Check sheet for the modelled part. Datum: model origin and axes. Units: mm. Face numbers are marked on the shaded views. Give positions to 0.01 mm unless a question says otherwise; leave off trailing zeros. Loops run counter-clockwise (first coordinate to the right, second up) from the corner with the lowest first, then second, coordinate; pieces in that order, holes last. Notation, with made-up numbers: M 42.5,4 L 87.5,4 A22 cw 87.5,40 Z; hole C 85,47 d8. An arc over 180 degrees is marked long. Use one line per item in the form item = value.
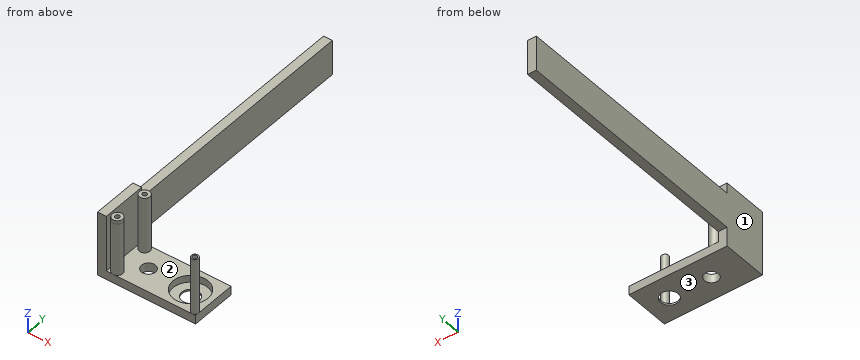
Autodesk Inventor part; units mm, degrees
ref_plane "YZ Plane" through (0, 0, 0) normal (1, 0, 0) x (0, 1, 0)
ref_plane "XZ Plane" through (0, 0, 0) normal (0, 1, 0) x (-1, 0, 0)
ref_plane "XY Plane" through (0, 0, 0) normal (0, 0, 1) x (1, 0, 0)
sketch "Sketch1" plane through (0, 0, 0) normal (0, 0, 1) x (1, 0, 0)
  line L0 (0, 0) -> (50.8, 0)
  line L1 (50.8, 0) -> (50.8, -33.02)
  line L2 (50.8, -33.02) -> (0, -33.02)
  line L3 (0, -33.02) -> (0, 0)
  dimension "d0" = 50.8
  dimension "d1" = 33.02
extrude "Extrusion1" add sketch "Sketch1" along normal blind 6.35
sketch "Sketch2" plane through (0, 0, 6.35) normal (0, 0, 1) x (1, 0, 0)
  line L0 (50.8, 0) -> (0, 0)
  line L1 (0, 0) -> (0, -33.02)
  circle A0 centre (34.29, -16.51) radius 12.7
  point P0 (7.62, -16.51)
  dimension "d4" = 16.51
  dimension "d5" = 16.51
  dimension "d6" = 26.67
  dimension "d7" = 7.62
  dimension "d8" = 25.4
extrude "Extrusion2" cut sketch "Sketch2" against normal blind 5.08
sketch "Sketch3" plane through (34.29, -16.51, 1.27) normal (0, 0, 1) x (1, 0, 0)
  circle A0 centre (0, 0) radius 6.35
  point P0 (-34.29, 16.51)
  dimension "d11" = 12.7
extrude "Extrusion3" cut sketch "Sketch3" against normal blind 5.08
sketch "Sketch14" plane through (0, -33.02, 0) normal (-1, 0, 0) x (0, 0, 1)
  line L0 (0, 33.02) -> (6.35, 33.02)
  line L1 (6.35, 33.02) -> (6.35, 0)
  line L2 (6.35, 0) -> (0, 0)
  line L3 (0, 0) -> (0, 33.02)
extrude "Extrusion14" add sketch "Sketch14" along normal blind 12.7
sketch "Sketch15" plane through (0, 0, 6.35) normal (0, 0, 1) x (1, 0, 0)
  line L0 (-12.7, -33.02) -> (-12.7, 0)
  line L1 (50.8, -33.02) -> (-12.7, -33.02)
  line L2 (50.8, 0) -> (-12.7, 0)
  circle A0 centre (-8.89, -3.81) radius 3.81
  circle A1 centre (-8.89, -29.21) radius 3.81
  circle A2 centre (-8.89, -29.21) radius 1.651
  circle A3 centre (-8.89, -3.81) radius 1.651
  point P0 (0, 0)
  dimension "d58" = 3.81
  dimension "d59" = 3.81
  dimension "d60" = 3.81
  dimension "d61" = 3.81
  dimension "d62" = 7.62
  dimension "d63" = 7.62
  dimension "d64" = 3.302
  dimension "d65" = 3.302
extrude "Extrusion15" add sketch "Sketch15" along normal blind 38.1 contours A1 | A0
sketch "Sketch16" plane through (0, 0, 6.35) normal (0, 0, 1) x (1, 0, 0)
  circle A0 centre (48.26, -30.48) radius 2.54
  line L0 (50.8, -33.02) -> (-8.89, -33.02)
  line L1 (50.8, -33.02) -> (50.8, 0)
  circle A1 centre (48.26, -30.48) radius 1.651
  point P0 (0, 0)
  dimension "d68" = 5.08
  dimension "d69" = 2.54
  dimension "d70" = 2.54
  dimension "d71" = 3.302
extrude "Extrusion16" add sketch "Sketch16" along normal blind 38.1 contours A0
sketch "Sketch17" plane through (-8.89, -3.81, 44.45) normal (0, 0, 1) x (1, 0, 0)
  circle A0 centre (0, 0) radius 1.651
  circle A1 centre (0, 0) radius 1.651
  circle A2 centre (0, 0) radius 3.81
  circle A3 centre (0, -25.396) radius 1.651
  circle A4 centre (0, -25.396) radius 3.81
  circle A5 centre (57.15, -26.67) radius 1.651
  circle A6 centre (57.15, -26.67) radius 1.651
  circle A7 centre (57.15, -26.67) radius 2.54
  point P0 (8.89, 3.81)
  dimension "d74" = 3.302
  dimension "d75" = 7.62
  dimension "d76" = 3.302
  dimension "d77" = 7.62
  dimension "d78" = 5.08
extrude "Extrusion17" add sketch "Sketch17" along normal blind 2.54
sketch "Sketch18" plane through (-12.7, -33.02, 0) normal (-1, 0, 0) x (0, 0, 1)
  line L0 (6.35, 3.81) -> (6.35, 0)
  line L1 (0, 33.02) -> (6.35, 33.02)
  line L2 (6.35, 33.02) -> (6.35, 0)
  line L3 (6.35, 0) -> (0, 0)
  line L4 (0, 0) -> (0, 33.02)
extrude "Extrusion18" add sketch "Sketch18" along normal blind 12.7
sketch "Sketch20" plane through (-25.4, -33.02, 0) normal (-1, 0, 0) x (0, 0, 1)
  line L0 (0, 33.02) -> (0, 0)
  line L1 (0, 0) -> (6.35, 0)
  line L2 (0, 33.02) -> (6.35, 33.02)
  line L3 (6.35, 33.02) -> (6.35, 0)
  line L4 (6.35, 0) -> (0, 0)
  line L5 (0, 0) -> (0, 33.02)
extrude "Extrusion20" cut sketch "Sketch20" against normal blind 5.08
sketch "Sketch21" plane through (0, 0, 6.35) normal (0, 0, 1) x (1, 0, 0)
  line L0 (-20.32, 0) -> (50.8, 0)
  line L1 (-20.32, 0) -> (-13.97, 0)
  line L2 (-13.97, 0) -> (-13.97, -33.02)
  line L3 (-13.97, -33.02) -> (-20.32, -33.02)
  line L4 (-20.32, -33.02) -> (-20.32, 0)
  point P0 (0, 0)
  dimension "d88" = 6.35
  dimension "d89" = 33.02
extrude "Extrusion21" add sketch "Sketch21" along normal blind 40.64
sketch "Sketch23" plane through (50.8, 0, 6.35) normal (0, 1, 0) x (1, 0, 0)
  line L0 (-64.77, 0) -> (-64.77, -40.64)
  line L1 (-64.77, -7.62) -> (-71.12, -7.62)
  line L2 (-71.12, -7.62) -> (-71.12, -33.02)
  line L3 (-71.12, -33.02) -> (-64.77, -33.02)
  line L4 (-64.77, -33.02) -> (-64.77, -7.62)
  line L5 (-64.77, -40.64) -> (-71.12, -40.64)
  point P0 (-50.8, 6.35)
  dimension "d94" = 25.4
  dimension "d95" = 6.35
  dimension "d96" = 7.62
extrude "Extrusion23" add sketch "Sketch23" along normal blind 177.8
sketch "Sketch24" plane through (0, 0, 6.35) normal (0, 0, 1) x (1, 0, 0)
  circle A0 centre (3.81, -16.51) radius 5.08
  circle A1 centre (34.29, -16.51) radius 6.35
  line L0 (48.26, -33.02) -> (-8.89, -33.02)
  point P0 (0, 0)
  dimension "d99" = 10.16
  dimension "d100" = 30.48
  dimension "d101" = 16.51
extrude "Extrusion24" cut sketch "Sketch24" against normal blind 25.4 contours A0
properties part number "servo attachment claw"
1) Section check A-A (x = 3.81). Record the cut outline in (y, z), then the cut area to 3 significant figures.
Evaluation:
outline = M -33.02,0 L -21.59,0 L -21.59,6.35 L -33.02,6.35 Z; M -11.43,0 L 0,0 L 0,6.35 L -11.43,6.35 Z
area = 145 mm^2
2) Scan lines: line 1 (X direction, y = -16, z = 3); line 2 (Y direction, x = 48.26, z = 16); line 3 (Y direction, x = -8, z = 45). Record each from-to range of solid material in increasing order.
Evaluation:
line_1 = -20.32 to -1.24, 8.86 to 21.6, 46.98 to 50.8
line_2 = -33.02 to -32.13, -28.83 to -27.94
line_3 = -32.91 to -30.6, -27.82 to -25.5, -7.51 to -5.2, -2.42 to -0.11
3) Section check B-B (z = 20.5). Record the cut outline in (x, y).
Evaluation:
outline = M -20.32,-33.02 L -13.97,-33.02 L -13.97,177.8 L -20.32,177.8 Z; C -8.89,-29.21 d7.62; C -8.89,-3.81 d7.62; C 48.26,-30.48 d5.08; hole C -8.89,-29.21 d3.3; hole C -8.89,-3.81 d3.3; hole C 48.26,-30.48 d3.3
4) Depth check by flat-ended pin: pin 1 Ø1 at (x, y) = (-9, -28.5) entering from +Z; pin 2 Ø8 at (x, y) = (3.81, -16.51) entering from +Z; pin 3 Ø5 at (x, y) = (-15.5, 63.5) entering from +Z; pin 4 Ø7 at (x, z) = (1, 9) entering from +Y. Enter the tip coordinate at first touch or a pass-through.
Evaluation:
pin_1 = 6.35
pin_2 = through
pin_3 = 39.37
pin_4 = 0
5) Release check for a two-part mould opening along X. For the marked faces 1, 2 and 3 record: pulls with the +X half, pulls with the -X half, needs draft (parallel to the pull), parting line crosses it, or undercut.
Evaluation:
face_1 = pulls with the -X half
face_2 = undercut
face_3 = needs draft
6) Section check C-C (y = -16.51). Record the cut outline in (x, z), then the cut area to 3 significant figures.
Evaluation:
outline = M -20.32,0 L -1.27,0 L -1.27,6.35 L -13.97,6.35 L -13.97,46.99 L -20.32,46.99 Z; M 8.89,0 L 27.94,0 L 27.94,1.27 L 21.59,1.27 L 21.59,6.35 L 8.89,6.35 Z; M 40.64,0 L 50.8,0 L 50.8,6.35 L 46.99,6.35 L 46.99,1.27 L 40.64,1.27 Z
area = 500 mm^2
